Model file for the job. Use its own axes, mm. A direction names the side the tool comes from. Give positions to 0.01 mm unless a question says otherwise; leave off trailing zeros. Write each loop counter-clockwise with the first axis right and the second up, starting at its lowest first coordinate (ties: lowest second). Pieces come first, ordered by that corner, then holes. Notation, with made-up numbers: (30.5, 5.5) - (58.5, 5.5) arc R21 ccw to (58.5, 23.5) - close; hole circle Ø11 at (82.5, -4.5). An arc over 180 degrees is marked (long way). Use CSV: the item, a comma, the result in double quotes.
Autodesk Inventor part; units mm, degrees
ref_plane "YZ Plane" through (0, 0, 0) normal (1, 0, 0) x (0, 1, 0)
ref_plane "XZ Plane" through (0, 0, 0) normal (0, 1, 0) x (-1, 0, 0)
ref_plane "XY Plane" through (0, 0, 0) normal (0, 0, 1) x (1, 0, 0)
sketch "Sketch1" plane through (0, 0, 0) normal (0, 1, 0) x (-1, 0, 0)
  line L0 (0, -6.9282) -> (-6, -3.4641)
  line L1 (-6, -3.4641) -> (-6, 3.4641)
  line L2 (-6, 3.4641) -> (0, 6.9282)
  line L3 (0, 6.9282) -> (6, 3.4641)
  line L4 (6, 3.4641) -> (6, -3.4641)
  line L5 (6, -3.4641) -> (0, -6.9282)
  point P0 (0, 0)
  point P1 (0, 0)
  dimension "d0" = 12
extrude "Extrusion1" add sketch "Sketch1" along normal blind 2.5
sketch "Sketch2" plane through (0, 2.5, 0) normal (0, 1, 0) x (1, 0, 0)
  circle A0 centre (0, 0) radius 2
  dimension "d3" = 4
extrude "Extrusion2" add sketch "Sketch2" along normal blind 15.8
thread "Thread1"
sketch "Sketch3" plane through (0, 0, 0) normal (0, -1, 0) x (1, 0, 0)
  circle A0 centre (0, 0) radius 5.5
  dimension "d8" = 11
extrude "Extrusion3" add sketch "Sketch3" along normal blind 3.44
sketch "Sketch4" plane through (0, -3.44, 0) normal (0, -1, 0) x (1, 0, 0)
  circle A0 centre (0, 0) radius 5.5
  circle A1 centre (0, 0) radius 5
  dimension "d11" = 10
extrude "Extrusion4" add sketch "Sketch4" along normal blind 16 contours A1
sketch "Sketch5" plane through (0, -19.44, 0) normal (0, -1, 0) x (1, 0, 0)
  circle A0 centre (0, 0) radius 5
  circle A1 centre (0, 0) radius 4
  dimension "d14" = 8
extrude "Extrusion5" cut sketch "Sketch5" against normal blind 10 contours A1
sketch "Sketch6" plane through (0, 0, 0) normal (1, 0, 0) x (0, 1, 0)
  circle A0 centre (-16.44, 0) radius 1
  line L0 (-19.44, -4) -> (-19.44, 4)
  point P0 (0, 0)
  dimension "d17" = 2
  dimension "d18" = 3
extrude "Extrusion6" cut sketch "Sketch6" along normal mid plane 14
sketch "Sketch7" plane through (0, 0, 0) normal (1, 0, 0) x (0, 1, 0)
  line L0 (2.5, -6.9282) -> (0, -6.9282) construction
  line L1 (0, -6.9282) -> (0, -5.5) construction
  line L2 (0, -5.5) -> (-3.44, -5.5) construction
  line L3 (-3.44, -5.5) -> (-3.44, -5) construction
  line L4 (-3.44, -5) -> (-19.44, -5) construction
  line L5 (-19.44, -5) -> (-19.44, -4) construction
  line L6 (-19.44, -4) -> (-9.44, -4) construction
  line L7 (-9.44, -4) -> (-9.44, 4) construction
  line L8 (-9.44, 4) -> (-19.44, 4) construction
  line L9 (-19.44, 4) -> (-19.44, 5) construction
  line L10 (-19.44, 5) -> (-3.44, 5) construction
  line L11 (-3.44, 5) -> (-3.44, 5.5) construction
  line L12 (-3.44, 5.5) -> (0, 5.5) construction
  line L13 (0, 5.5) -> (0, 6.9282) construction
  line L14 (0, 6.9282) -> (2.5, 6.9282) construction
  line L15 (2.5, 6.9282) -> (2.5, 2) construction
  line L16 (2.5, 2) -> (18.3, 2) construction
  line L17 (18.3, 2) -> (18.3, -2) construction
  line L18 (18.3, -2) -> (2.5, -2) construction
  line L19 (2.5, -2) -> (2.5, -6.9282) construction
  circle A0 centre (-18.84, 5) radius 0.3
  line L20 (-19.44, -4) -> (-19.44, 4)
  line L21 (-26.988, 0) -> (25.848, 0)
  point P0 (0, 0)
  dimension "d21" = 0.6
  dimension "d22" = 0.6
revolve "Revolution1" cut sketch "Sketch7" angle 360 about axis through (0, -10, 0) along (0, 1, 0)
sketch "Sketch8" plane through (0, 0, 0) normal (0, 0, 1) x (1, 0, 0)
  line L0 (-5.078, 3.1229) -> (-8.0424, 0.1585)
  line L1 (-8.0424, 0.1585) -> (-8.4208, 3.1229)
  line L2 (-8.4208, 3.1229) -> (-5.078, 3.1229)
  line L3 (-6, 2.5) -> (0, 2.5)
  line L4 (0, -26.988) -> (0, 25.848)
  point P0 (0, 0)
  dimension "d24" = 45
revolve "Revolution2" cut sketch "Sketch8" angle 360 about axis through (0, -10, 0) along (0, 1, 0)
properties part number "500-126" material "Steel"
(1) Pull direction Z, two halves, no side cores. Call faces 4 (the face through (4.429, -15.486, -0.3)), 5 (the face through (0, 0, -6)), 6 (the face through (-1.08, -19.29, 4.88)): released by +Z, released by -Z, zero draft, split by the parting line, or undercut.
Checked values:
face 4,"undercut"
face 5,"zero draft"
face 6,"split by the parting line"
(2) Saw through at C-C, the plane y = 7.5. List the corners of the cut face in (x, z), then the cut area to 3 significant figures.
Checked values:
outline,"circle Ø4 at (0, 0)"
area,"12.6 mm^2"
(3) Saw through at A-A, the plane z = 0. Count the separate pieces of the cut face and the enclosed holes in it, then the cut area to 3 significant figures.
Checked values:
separate pieces,"3"
enclosed holes,"0"
area,"207 mm^2"
(4) Flat gauge pins, fed straight in: P1, Ø2.5, axis at y = -16.44, z = 0, coming from the -X side; P2, Ø5, axis at x = 1.5, y = -10.5, coming from the -Z side; P3, Ø6, axis at y = -7, z = -2.5, coming from the +X side; P4, Ø1.2, axis at y = -16.44, z = 0, coming from the -X side. Where does each tip first touch, or does it go through?
Checked values:
P1,"stops at x = -5"
P2,"stops at z = -5"
P3,"stops at x = 5"
P4,"passes through"
(5) Saw through at B-B, the plane y = -16.44. List the corners of the cut face in (x, z).
Checked values:
outline,"(-4.9, -1) arc R5 ccw to (4.9, -1) - (3.87, -1) arc R4 cw to (-3.87, -1) - close; (-4.9, 1) - (-3.87, 1) arc R4 cw to (3.87, 1) - (4.9, 1) arc R5 ccw to start"
(6) Wall check: probe 1 along Y at (x, z) = (4.65, 0); probe 2 along X at (y, z) = (-11.25, 0); probe 3 along Y at (x, z) = (4.25, -0.5). Give the ranges that are in metal, low to high. Write a range as [from, to].
Checked values:
probe 1,"y = [-19.44, -17.44], [-15.44, 2.5]"
probe 2,"x = [-5, -4], [4, 5]"
probe 3,"y = [-19.44, -17.31], [-15.57, 2.5]"
(7) 3-axis set-ups, long thin cutter, end or side, ignore diameter. For faces 1 (the face through (3.042, 0.841, 5.172)), 2 (the face through (-2.5, 2.5, 0.1)), 3 (the face through (4.77, -10.88, -1.5)): which of +Z, -Z, +X, -X, +Y, -Y reach the whole face in a straight line?
Checked values:
face 1,"+Z, +X, +Y, -Y"
face 2,"+Y"
face 3,"-Y"
